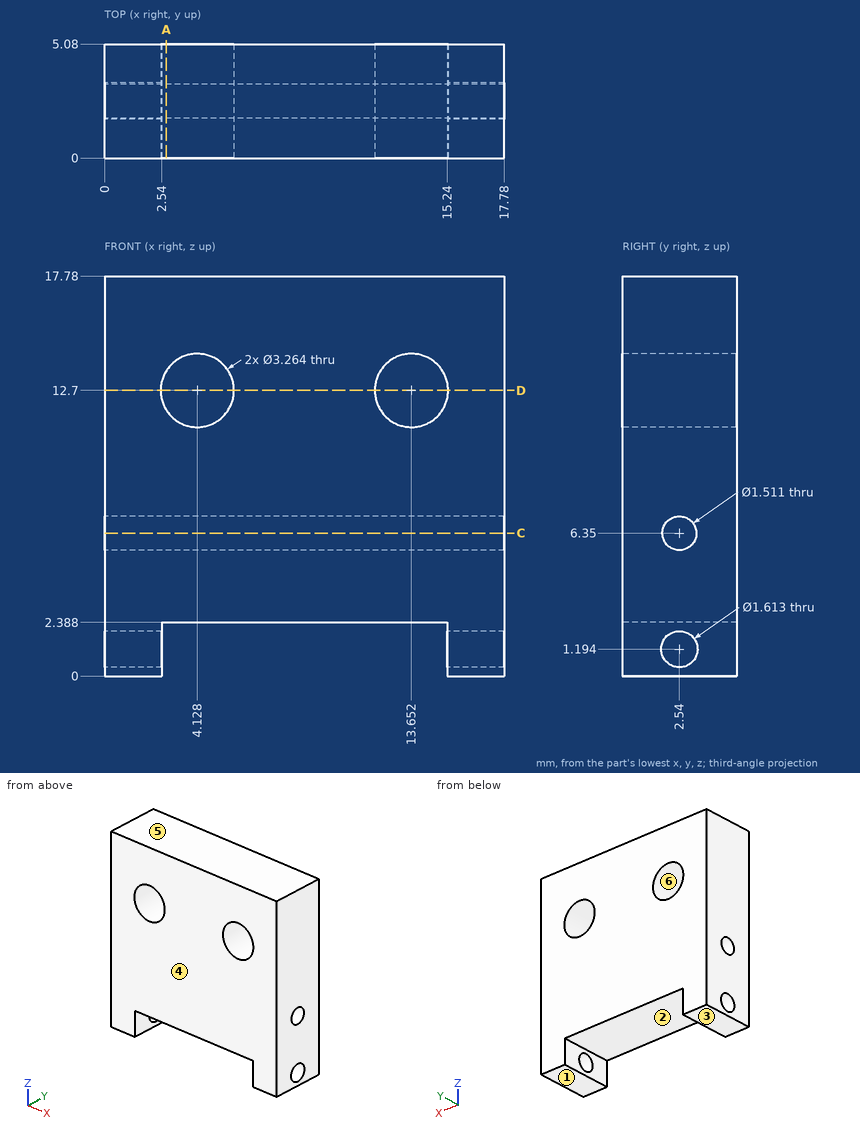
Geometry: see drawing. Coordinates: mm, zero at the bounding-box minimum. A direction names the side the tool comes from. Round coordinates to 2 decimals unless told otherwise and drop trailing zeros. Write each loop counter-clockwise with the first axis right and the second up, starting at its lowest first coordinate (ties: lowest second). Pieces come first, ordered by that corner, then holes.
Item 1: Set-up query: the marked faces 1 and 2. Return all of +Z, -Z, +X, -X, +Y, -Y with unobstructed straight access to the full face (end or side cutting, diameter ignored); none if empty.
Item 2: Section query A-A (x = 2.75). Give the number of separate pieces and of enclosed holes in the cut face.
Item 3: Pin query (flat end, axial travel): P1, Ø1.5, axis at x = 5, y = 4, coming from the -Z side. Return the tip coordinate at first contact, or that it passes through.
Item 4: Section query C-C (z = 6.35). Return loops of the section in (x, y) (1 decimal).
Item 5: Mould query, pull axis Z, two halves, no side actions, for the marked faces 3, 4, 5 and 6. Classes: +Z half, -Z half, draft (parallel to the pull), parting line (faces both ways), or undercut.
Item 6: Section query D-D (z = 12.7). Return loops of the section in (x, y) (1 decimal).
Item 7: Material intervals for L1, parallel to Z at x = 12.5, y = 2.9 (1 decimal); L2, parallel to X at y = 3.4, z = 1.5; L3, parallel to Z at x = 13.5, y = 2.3 (1 decimal), sorted ascending.
Completed:
1. face 1: -Z, +X, -X, +Y, -Y
1. face 2: -Z, +Y, -Y
2. separate pieces: 2
2. enclosed holes: 1
3. P1: stops at z = 2.39
4. outline: (0, 0) - (17.8, 0) - (17.8, 1.8) - (0, 1.8) - close; (0, 3.3) - (17.8, 3.3) - (17.8, 5.1) - (0, 5.1) - close
5. face 3: -Z half
5. face 4: draft
5. face 5: +Z half
5. face 6: undercut
6. outline: (0, 0) - (2.5, 0) - (2.5, 5.1) - (0, 5.1) - close; (5.8, 0) - (12, 0) - (12, 5.1) - (5.8, 5.1) - close; (15.3, 0) - (17.8, 0) - (17.8, 5.1) - (15.3, 5.1) - close
7. L1: z = 2.4 to 5.7, 7 to 11.5, 13.9 to 17.8
7. L2: x = 0 to 2.54, 15.24 to 17.78
7. L3: z = 2.4 to 5.6, 7.1 to 11.1, 14.3 to 17.8
